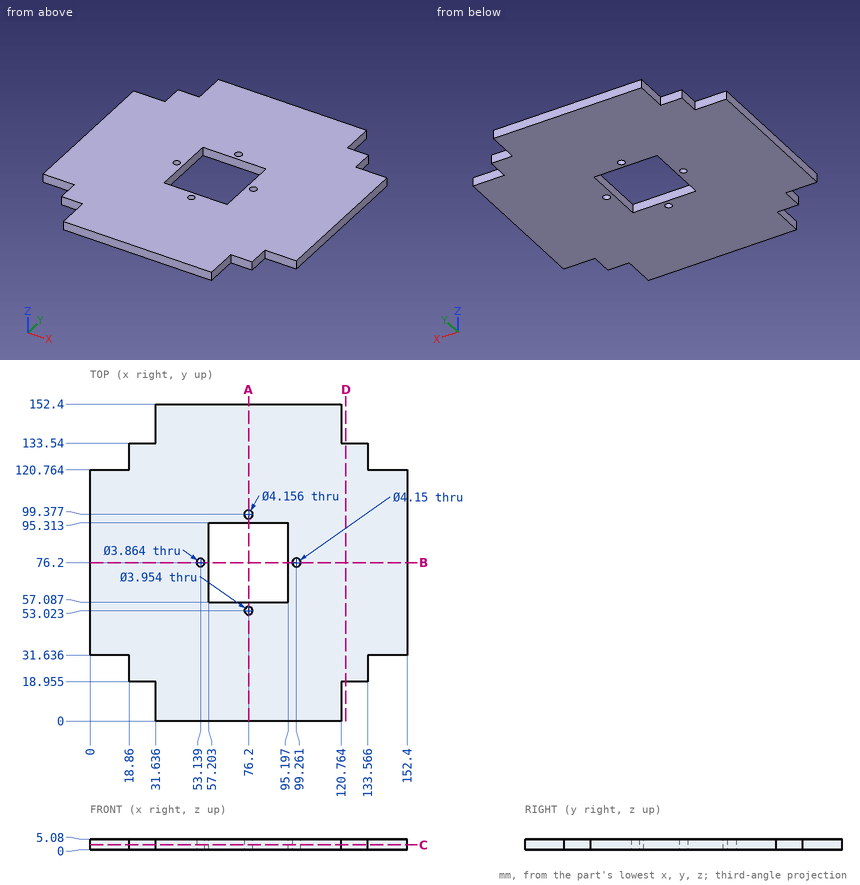
Could you check a few things on this drawing? It's one solid part, dimensions in mm from its lowest x, y, z. Coordinates: 2 decimals unless noted, no trailing zeros. Write each loop counter-clockwise with the first axis right and the second up, starting at its lowest first coordinate (ties: lowest second). Pieces come first, ordered by that corner, then holes. Notation, with made-up numbers: (36, 19) - (48, 19) arc R24 ccw to (48, 33) - close; hole circle Ø2 at (-9, -17). An arc over 180 degrees is marked (long way). Use one line per item in the form item = value.
1) Suppose I cut it at D-D, the plane x = 123. Write out the boundary of the cut face in (y, z) (1 decimal), plus the area to 3 significant figures.
Solved:
outline = (19, 0) - (133.5, 0) - (133.5, 5.1) - (19, 5.1) - close
area = 582 mm2
2) Suppose I cut it at C-C, the plane z = 2.3. Give the number of separate pieces and of enclosed holes in the cut face, plus the area to 3 significant figures.
Solved:
separate_pieces = 1
enclosed_holes = 5
area = 18,400 mm2
3) Suppose I cut it at B-B, the plane y = 76.2. Write out the boundary of the cut face in (x, z) (1 decimal).
Solved:
outline = (0, 0) - (51.2, 0) - (51.2, 5.1) - (0, 5.1) - close; (55.1, 0) - (57.2, 0) - (57.2, 5.1) - (55.1, 5.1) - close; (95.2, 0) - (97.2, 0) - (97.2, 5.1) - (95.2, 5.1) - close; (101.3, 0) - (152.4, 0) - (152.4, 5.1) - (101.3, 5.1) - close
4) I'm going to push flat-ended pins straight in: P1, Ø2.5, axis at x = 6.5, z = 2.5, coming from the +Y side; P2, Ø3.5, axis at x = 53.14, y = 76.2, coming from the +Z side. Where does each tip first touch, or does it pass through?
Solved:
P1 = 120.76
P2 = through
5) Suppose I cut it at A-A, the plane x = 76.2. Write out the boundary of the cut face in (y, z) (1 decimal), plus the area to 3 significant figures.
Solved:
outline = (0, 0) - (51, 0) - (51, 5.1) - (0, 5.1) - close; (55, 0) - (57.1, 0) - (57.1, 5.1) - (55, 5.1) - close; (95.3, 0) - (97.3, 0) - (97.3, 5.1) - (95.3, 5.1) - close; (101.5, 0) - (152.4, 0) - (152.4, 5.1) - (101.5, 5.1) - close
area = 539 mm2
6) I need wall thicknesses on line 1 (Y direction, x = 76.2, z = 2.4) (1 decimal); line 2 (Y direction, x = 80, z = 3.5); line 3 (X direction, y = 81.5, z = 3.65). Which ranges of each line are inside material? Lowest first, please.
Solved:
line_1 = 0 to 51, 55 to 57.1, 95.3 to 97.3, 101.5 to 152.4
line_2 = 0 to 57.09, 95.31 to 152.4
line_3 = 0 to 57.2, 95.2 to 152.4
